Can you work these out from the drawing? Everything is in mm from the part's minimum corner. Coordinates: 2 decimals unless noted, no trailing zeros. Order: outer loops, then holes, each group sorted by start corner. A loop starts at its lowest first (then second) coordinate and runs counter-clockwise, first axis right, second up. Notation, with made-up numbers: (65.5, 66) -> (109.5, 66) arc R17 ccw to (109.5, 76) -> close; hole circle Ø6 at (39, 40.5). An arc over 180 degrees is marked (long way). Return JSON: item names as keys, results as strings. Group by question number.
1) If we section it at A-A, the plane y = 3: Please give me the cut outline in (x, z).
2) If we section it at D-D, the plane z = 27.75: Please give me the cut outline in (x, y).
3) If we section it at B-B, the plane x = 55: Please give me the cut outline in (y, z).
4) If we section it at C-C, the plane z = 7.25: Please give me the cut outline in (x, y).
5) For pin 1 (7 mm diameter, centred on x = 55, z = 27.75, fed in from +Y); pin 2 (1.2 mm diameter, centred on y = 1.5, z = 27.5, fed in from +X); pin 3 (2 mm diameter, centred on x = 29, y = 1.5, fed in from +Z), each with a flat end and sliding along its axis, tell me the tip position at first contact or that it passes through.
6) If I drill on probe 1 along Z at (x, y) = (55, 0.5); probe 2 along X at (y, z) = (0.7, 7.25); probe 3 along X at (y, z) = (0.4, 27.75), over which ranges is the centre line in solid material (lowest first)? Write a range as from..to.
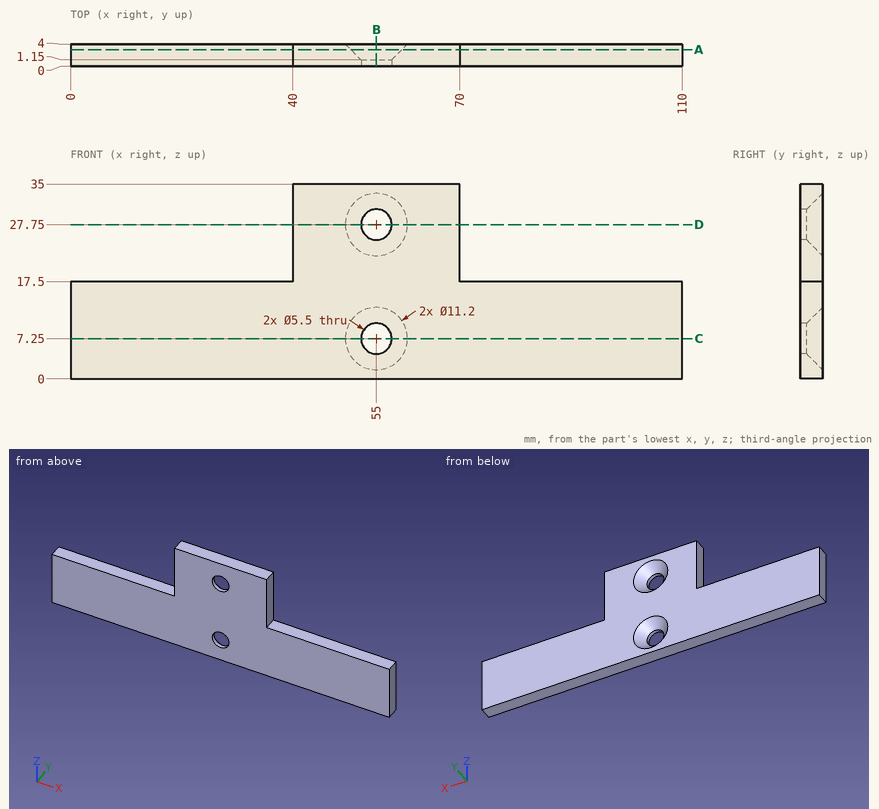
Result sheet:
{
 "1": {"outline": "(0, 0) -> (110, 0) -> (110, 17.5) -> (70, 17.5) -> (70, 35) -> (40, 35) -> (40, 17.5) -> (0, 17.5) -> close; hole circle Ø9.2 at (55, 7.25); hole circle Ø9.2 at (55, 27.75)"},
 "2": {"outline": "(40, 0) -> (52.25, 0) -> (52.25, 1.15) -> (49.4, 4) -> (40, 4) -> close; (57.75, 0) -> (70, 0) -> (70, 4) -> (60.6, 4) -> (57.75, 1.15) -> close"},
 "3": {"outline": "(0, 0) -> (4, 0) -> (4, 1.65) -> (1.15, 4.5) -> (0, 4.5) -> close; (0, 10) -> (1.15, 10) -> (4, 12.85) -> (4, 22.15) -> (1.15, 25) -> (0, 25) -> close; (0, 30.5) -> (1.15, 30.5) -> (4, 33.35) -> (4, 35) -> (0, 35) -> close"},
 "4": {"outline": "(0, 0) -> (52.25, 0) -> (52.25, 1.15) -> (49.4, 4) -> (0, 4) -> close; (57.75, 0) -> (110, 0) -> (110, 4) -> (60.6, 4) -> (57.75, 1.15) -> close"},
 "5": {"pin 1": "stops at y = 1.9", "pin 2": "stops at x = 70", "pin 3": "stops at z = 17.5"},
 "6": {"probe 1": "z = 0..4.5, 10..25, 30.5..35", "probe 2": "x = 0..52.25, 57.75..110", "probe 3": "x = 40..52.25, 57.75..70"}
}
